Autodesk Inventor part; units mm, degrees
ref_plane "YZ Plane" through (0, 0, 0) normal (1, 0, 0) x (0, 1, 0)
ref_plane "XZ Plane" through (0, 0, 0) normal (0, 1, 0) x (-1, 0, 0)
ref_plane "XY Plane" through (0, 0, 0) normal (0, 0, 1) x (1, 0, 0)
sketch "Sketch1" plane through (0, 0, 0) normal (0, 0, 1) x (1, 0, 0)
  arc A0 (2.6458, 3) -> (2.6458, -3) centre (0, 0) ccw
  arc A1 (4, 3) -> (4, -3) centre (0, 0) ccw
  line L0 (-4, -3) -> (-11, -3)
  line L1 (-11, -3) -> (-11, 3)
  line L2 (-11, 3) -> (-4, 3)
  line L3 (-4, 3) -> (-4, -3)
  line L4 (2.6458, 3) -> (4, 3)
  line L5 (4, 3) -> (4, -3) construction
  line L6 (4, -3) -> (2.6458, -3)
  line L7 (2.6458, -3) -> (2.6458, 3) construction
  line L8 (-11, 3) -> (-3, 3)
  line L9 (-3, 3) -> (-3, 4)
  line L10 (-3, 4) -> (-11, 4)
  line L11 (-11, 4) -> (-11, 3)
  line L12 (-11, -3) -> (-3, -3)
  line L13 (-3, -3) -> (-3, -4)
  line L14 (-3, -4) -> (-11, -4)
  line L15 (-11, -4) -> (-11, -3)
  point P0 (2.6458, 0)
  dimension "d0" = 8
  dimension "d1" = 10
  dimension "d3" = 6
  dimension "d24" = 11
  dimension "d25" = 1
  dimension "d26" = 1
extrude "Extrusion1" add sketch "Sketch1" along normal blind 30
sketch "Sketch2" plane through (-11, -4, 0) normal (-1, 0, 0) x (0, 0, 1)
  circle A0 centre (8, 4) radius 1.5
  circle A1 centre (26, 4) radius 1.5
  line L0 (0, 8) -> (0, 0)
  point P0 (0, 4)
  dimension "d6" = 3
  dimension "d9" = 3
  dimension "d10" = 18
extrude "Extrusion2" cut sketch "Sketch2" against normal blind 10
fillet "Fillet1" radius 0.5 2 edges at (4, 3, 15) (4, -3, 15)
sketch "Sketch3" plane through (-11, -4, 0) normal (0, -1, 0) x (1, 0, 0)
  circle A0 centre (3.5, 15) radius 2.5
  line L0 (0, 0) -> (0, 30)
  line L1 (0, 0) -> (7, 0)
  line L2 (19.5327, 37.0698) -> (11.5, 15)
  line L3 (19.5327, 37.0698) -> (43.0189, 37.0698) construction
  line L4 (11.5, 15) -> (19.5327, 1.0869)
  line L5 (19.5327, 1.0869) -> (19.5327, 37.0698)
  point P0 (11, 0)
  point P1 (0, 15)
  point P2 (3.5, 0)
  dimension "d14" = 5
  dimension "d17" = 110
  dimension "d18" = 130
  dimension "d19" = 8
extrude "Extrusion3" cut sketch "Sketch3" along normal through all both and the other way through all
sketch "Sketch4" plane through (0, 0, 0) normal (1, 0, 0) x (0, 1, 0)
  spline S0 degree 2 poles (0, 9.5) (2.5981, 9.5) (1.299, 7.25) (0, 5) (-1.299, 7.25) (-2.5981, 9.5) (0, 9.5) knots 0 0 0 0.333333 0.333333 0.666667 0.666667 1 1 1 weights 1 0.5 1 0.5 1 0.5 1
  spline S1 degree 2 poles (0, 27.5) (2.5981, 27.5) (1.299, 25.25) (0, 23) (-1.299, 25.25) (-2.5981, 27.5) (0, 27.5) knots 0 0 0 0.333333 0.333333 0.666667 0.666667 1 1 1 weights 1 0.5 1 0.5 1 0.5 1
  circle A0 centre (0, 26) radius 2.5
  circle A1 centre (0, 8) radius 2.5
  point P0 (0, 0)
  dimension "d20" = 5
  dimension "d21" = 5
extrude "Extrusion4" cut sketch "Sketch4" against normal blind 7
equation "\"d26\" = d25"
properties part number "brush clip"
Verification items for the finished model (mm, model axes). A direction names the side the tool comes from. Coordinates: 2 decimals unless noted, no trailing zeros. Order: outer loops, then holes, each group sorted by start corner. A loop starts at its lowest first (then second) coordinate and runs counter-clockwise, first axis right, second up. Notation, with made-up numbers: M 85,64.25 L 92,64.25 A10 cw 92,75.25 Z; hole C 76.5,-16 d11. An arc over 180 degrees is marked long. One line per item, written item: value. Start each with the question number.
Item 1: Sectioned sample at A-A (y = 0). Enter the section's corners in (x, z).
Item 2: Sectioned sample at B-B (x = 0). Enter the section's corners in (y, z).
Item 3: Mould release check, pull along Y, two halves, no side actions. Record for faces 4 (the cylindrical face through (3.303, -3.341, 25.759)), 5 (the flat face through (-11, 0, 15)), 6 (the flat face through (-4, 4, 15)): released by +Y, released by -Y, zero draft, split by the parting line, or undercut.
Item 4: Sectioned sample at C-C (x = -7.5). Enter the section's corners in (y, z).
Item 5: Scan lines: probe 1 along Y at (x, z) = (0, 22); probe 2 along Z at (x, y) = (-4.25, -2); probe 3 along Z at (x, y) = (-5.5, 1). Record each from-to range of solid material in increasing order.
Item 6: Sectioned sample at D-D (z = 16). Enter the section's corners in (x, y).
Item 7: Gauge pin test, flat ends, axial feed: pin 1 (1 mm diameter, centred on x = 1.5, z = 3.5, fed in from -Y); pin 2 (5 mm diameter, centred on y = 3.5, z = 19.5, fed in from +X); pin 3 (5.5 mm diameter, centred on y = 0, z = 7, fed in from +X); pin 4 (2.5 mm diameter, centred on y = 0, z = 8, fed in from +X). Record the tip position at first contact, or that the pin passes through.
Item 8: Access from +Z, -Z, +X, -X, +Y, -Y to the whole of each face (thin tool, end or side, straight path). Record for faces 1 (the flat face through (1.934, -3.974, 18.94)), 2 (the cylindrical face through (-5.465, 2.385, 26.751)), 3 (the flat face through (-4, -4, 15)).
Conclusion:
1. outline: M -11,0 L -4,0 L -4,5.5 L -7,5.5 L -7,6.5 L -11,6.5 Z; M -11,9.5 L -7,9.5 L -7,10.5 L -4,10.5 L -4,23.5 L -7,23.5 L -7,24.5 L -11,24.5 Z; M -11,27.5 L -7,27.5 L -7,28.5 L -4,28.5 L -4,30 L -11,30 Z; hole C -7.5,15 d5
2. outline: M -5,0 L -4,0 L -4,30 L -5,30 Z; M 4,0 L 5,0 L 5,30 L 4,30 Z
3. face 4: undercut
3. face 5: zero draft
3. face 6: released by +Y
4. outline: M -4,0 L 4,0 L 4,12.5 L -4,12.5 Z; M -4,17.5 L 4,17.5 L 4,30 L -4,30 Z; hole C 0,8 d3; hole C 0,26 d3
5. probe 1: y = -5 to -4, 4 to 5
5. probe 2: z = 0 to 6.5, 9.5 to 24.5, 27.5 to 30
5. probe 3: z = 0 to 5.71, 10.29 to 13.5, 16.5 to 23.71, 28.29 to 30
6. outline: M -11,-4 L -9.79,-4 L -9.79,4 L -11,4 Z; M -5.21,-4 L -3,-4 A5 ccw 0.86,-4.92 L 0.86,-3.91 A4 cw long 0.86,3.91 L 0.86,4.92 A5 ccw -3,4 L -5.21,4 Z
7. pin 1: stops at y = -4.9
7. pin 2: stops at x = 3.05
7. pin 3: stops at x = -2.9
7. pin 4: passes through
8. face 1: +X, +Y, -Y
8. face 2: +X
8. face 3: +Z, -Z, -X, -Y
